from build123d import *

# Parameters (mm, degrees)
BOSS_EXTRUDE1_DEPTH = 2.8
CUT_EXTRUDE1_DEPTH  = 0.5
SKETCH3_R           = 2
BOSS_EXTRUDE2_DEPTH = 25


with BuildPart() as part:
    # Sketch1 → Boss-Extrude1 (new body)
    with BuildSketch(Plane(origin=(0, 0, 0), x_dir=(1, 0, 0), z_dir=(0, 1, 0))):
        Polygon((1.957217413, -3.39), (3.914434825, 0), (1.957217413, 3.39), (-1.957217413, 3.39), (-3.914434825, 0), (-1.957217413, -3.39), align=None)
    extrude(amount=BOSS_EXTRUDE1_DEPTH)

    # Sketch2 → Cut-Extrude1 (cut)
    with BuildSketch(Plane(origin=(0, 2.8, 0), x_dir=(1, 0, 0), z_dir=(0, 1, 0))):
        Polygon((-0.5, 3.39), (0.5, 3.39), (0.5, 0.5), (3.914434825, 0.5), (3.914434825, -0.5), (0.5, -0.5), (0.5, -3.39), (-0.5, -3.39), (-0.5, -0.5), (-3.914434825, -0.5), (-3.914434825, 0.5), (-0.5, 0.5), align=None)
    extrude(amount=-CUT_EXTRUDE1_DEPTH, mode=Mode.SUBTRACT)

    # Sketch3 → Boss-Extrude2 (add)
    with BuildSketch(Plane.XZ):
        with Locations(Location((0, 0, 0), (0, 0, 270))):
            Circle(SKETCH3_R)
    extrude(amount=BOSS_EXTRUDE2_DEPTH)


solid = part.part
Geometry: final body of the model. Coordinates: model frame, mm. A direction names the side the tool comes from. Round coordinates to 2 decimals unless told otherwise and drop trailing zeros. Order: outer loops, then holes, each group sorted by start corner. A loop starts at its lowest first (then second) coordinate and runs counter-clockwise, first axis right, second up. Notation, with made-up numbers: (3, 81.5) -> (44, 81.5) arc R8 ccw to (44, 95.5) -> close; hole circle Ø6 at (75.5, -40). An arc over 180 degrees is marked (long way). Put each result on its own line as item: value. Start each with the question number.
Q1. First-contact query: pin 1 (1.5 mm diameter, centred on x = 0, z = 2.5, fed in from +Y); pin 2 (1.5 mm diameter, centred on x = -2.5, y = -2, fed in from +Z); pin 3 (2 mm diameter, centred on y = -21, z = 2, fed in from -X). Flat tips, straight axial feed; report the tip coordinate or a pass-through.
Q2. Section A-A on x = 0. Return the cut outline in (y, z), and give its area (3 significant figures).
Q3. Line query: probe 1 along Y at (x, z) = (-2, 3); probe 2 along Y at (x, z) = (0, 3); probe 3 along Z at (x, y) = (1, -21). Output: solid intervals per line, ascending.
Q4. Pull-direction query (X, two-part tool) for faces 1 (the flat face through (0, 2.3, 0)), 2 (the flat face through (2.95, 1.38, -1.67)), 3 (the flat face through (-2.95, 1.38, 1.67)); classes: +X half, -X half, draft (parallel to the pull), parting line (faces both ways), or undercut.
Q5. Reachability of faces 4 (the flat face through (2, 0, -2)), 5 (the flat face through (2.92, 1.38, 1.72)) from +Z, -Z, +X, -X, +Y, -Y: full face, straight path, thin tool, end or side. Return the list, or none.
Q6. Section D-D on x = -2.75. Return the cut outline in (y, z), and give its area (3 significant figures).
Q7. Section C-C on y = -12.75. Return the cut outline in (x, z).
Q8. Section B-B on z = 1.25. Return the cut outline in (x, y).
Ans:
1. pin 1: stops at y = 2.8
1. pin 2: stops at z = 0.97
1. pin 3: stops at x = -1.73
2. outline: (-25, -2) -> (0, -2) -> (0, -3.39) -> (2.3, -3.39) -> (2.3, 3.39) -> (0, 3.39) -> (0, 2) -> (-25, 2) -> close
2. area: 116 mm2
3. probe 1: y = 0 to 2.8
3. probe 2: y = 0 to 2.3
3. probe 3: z = -1.73 to 1.73
4. face 1: undercut
4. face 2: +X half
4. face 3: -X half
5. face 4: -Y
5. face 5: +Z, +X, +Y, -Y
6. outline: (0, -2.02) -> (2.8, -2.02) -> (2.8, -0.5) -> (2.3, -0.5) -> (2.3, 0.5) -> (2.8, 0.5) -> (2.8, 2.02) -> (0, 2.02) -> close
6. area: 10.8 mm2
7. outline: circle Ø4 at (0, 0)
8. outline: (-3.19, 0) -> (-1.56, 0) -> (-1.56, -25) -> (1.56, -25) -> (1.56, 0) -> (3.19, 0) -> (3.19, 2.8) -> (0.5, 2.8) -> (0.5, 2.3) -> (-0.5, 2.3) -> (-0.5, 2.8) -> (-3.19, 2.8) -> close
